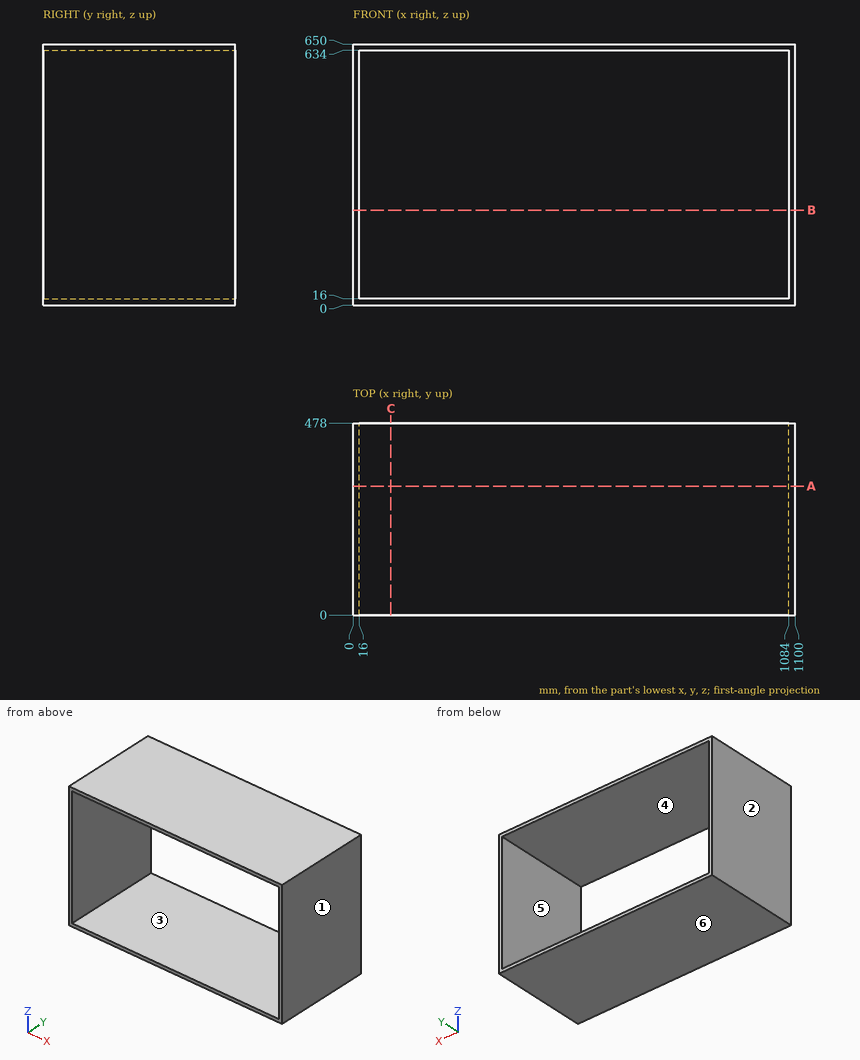
Geometry: see drawing. Coordinates: mm, zero at the bounding-box minimum. A direction names the side the tool comes from. Give positions to 0.01 mm unless a question says otherwise; leave off trailing zeros. Loops run counter-clockwise (first coordinate to the right, second up) from the corner with the lowest first, then second, coordinate; pieces in that order, holes last. Notation, with made-up numbers: (33, 47.5) -> (78, 47.5) arc R36 ccw to (78, 84.5) -> close; hole circle Ø10 at (74.5, 77). An arc over 180 degrees is marked (long way). Answer as a JSON object with one key per item and string values. Group by question number.
Item 1: Cut plane A-A, the plane y = 321.5. Return the cut outline in (x, z).
Item 2: Pull-direction query (X, two-part tool) for the marked faces 1, 2, 3 and 4; classes: released by +X, released by -X, zero draft, split by the parting line, or undercut.
Item 3: Line query: probe 1 along X at (y, z) = (60.5, 424); probe 2 along Z at (x, y) = (820, 79). Output: solid intervals per line, ascending.
Item 4: Reachability of the marked faces 5 and 6 from +Z, -Z, +X, -X, +Y, -Y: full face, straight path, thin tool, end or side. Return the list, or none.
Item 5: Cut plane B-B, the plane z = 236.5. Return the cut outline in (x, y), and give its area (3 significant figures).
Item 6: Cut plane C-C, the plane x = 94. Return the cut outline in (y, z).
Checks:
{
 "1": {"outline": "(0, 0) -> (1100, 0) -> (1100, 650) -> (0, 650) -> close; hole (16, 16) -> (1084, 16) -> (1084, 634) -> (16, 634) -> close"},
 "2": {"face 1": "released by +X", "face 2": "released by -X", "face 3": "undercut", "face 4": "undercut"},
 "3": {"probe 1": "x = 0 to 16, 1084 to 1100", "probe 2": "z = 0 to 16, 634 to 650"},
 "4": {"face 5": "+Y, -Y", "face 6": "-Z, +X, -X, +Y, -Y"},
 "5": {"outline": "(0, 0) -> (16, 0) -> (16, 478) -> (0, 478) -> close; (1084, 0) -> (1100, 0) -> (1100, 478) -> (1084, 478) -> close", "area": "15,300 mm²"},
 "6": {"outline": "(0, 0) -> (478, 0) -> (478, 16) -> (0, 16) -> close; (0, 634) -> (478, 634) -> (478, 650) -> (0, 650) -> close"}
}
